Read the model definition and answer for the solid it produces. Units are mm, in the model's axes. Give positions to 0.01 mm unless a question says otherwise; leave off trailing zeros. Loops run counter-clockwise (first coordinate to the right, second up) from the corner with the lowest first, then second, coordinate; pieces in that order, holes last. Notation, with made-up numbers: (2, 76.5) -> (51, 76.5) arc R26 ccw to (51, 100.5) -> close; hole circle Ø5 at (-0.75, -32.75). An arc over 180 degrees is marked (long way). Answer as CSV lines item,"result". Start each with the question number.
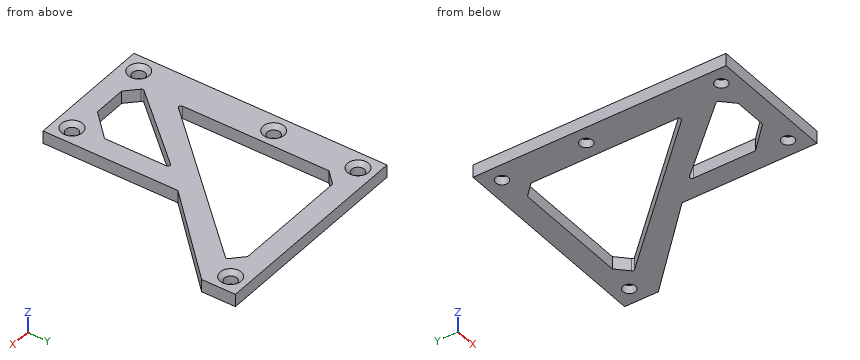
```python
from build123d import *

# Parameters (mm, degrees)
PAD_DEPTH    = 3
SKETCH001_R  = 1.5
POCKET_DEPTH = 5
FILLET_R     = 0.5
FILLET001_R  = 0.5
CHAMFER_SIZE = 1


with BuildPart() as part:
    # Sketch → Pad (new body)
    with BuildSketch(Plane.XY):
        Polygon((0, 0), (0, -60), (8, -60), (30, -60), (30, -28), (50, -8), (50, 0), align=None)
        Polygon((8, -8), (11, -5), (39, -5), (42, -8), (8, -44), align=None, mode=Mode.SUBTRACT)
        Polygon((8, -52), (25, -33), (25, -49), (19, -55), (11, -55), align=None, mode=Mode.SUBTRACT)
    extrude(amount=PAD_DEPTH)

    # Sketch001 (on Face19 of Pad) → Pocket (cut)
    with BuildSketch(Plane.XY.offset(3)):
        with Locations((4, -4)):
            Circle(SKETCH001_R)
        with Locations((46, -4)):
            Circle(SKETCH001_R)
        with Locations((4, -24)):
            Circle(SKETCH001_R)
        with Locations((4, -56)):
            Circle(SKETCH001_R)
        with Locations((26, -56)):
            Circle(SKETCH001_R)
    extrude(amount=-POCKET_DEPTH, mode=Mode.SUBTRACT)

    # Fillet
    fillet_edges = [part.edges().sort_by_distance(p)[0] for p in [
        (8, -44, 1.5),
        (25, -33, 1.5),
    ]]
    fillet(fillet_edges, radius=FILLET_R)

    # Fillet001
    fillet001_edges = [part.edges().sort_by_distance(p)[0] for p in [
        (8, -52, 1.5),
        (42, -8, 1.5),
    ]]
    fillet(fillet001_edges, radius=FILLET001_R)

    # Chamfer
    chamfer_edges = [part.edges().sort_by_distance(p)[0] for p in [
        (2.5, -4, 3),
        (2.5, -24, 3),
        (2.5, -56, 3),
        (24.5, -56, 3),
        (44.5, -4, 3),
    ]]
    chamfer(chamfer_edges, length=CHAMFER_SIZE)


solid = part.part
```
(1) Find section A-A on x = 4. Write down the section's boundary in (y, z), then the cut area to 3 significant figures.
(2) Find section C-C on y = -29. Write down the section's boundary in (x, z).
(3) Find section D-D on z = 2.45. Write down the section's boundary in (x, y), then the cut area to 3 significant figures.
(4) Find section B-B on x = 26. Write down the section's boundary in (y, z), then the cut area to 3 significant figures.
(5) Each of these flat-tipped pins is pushed along its axis until it touches: P1, Ø0.9, axis at y = -21, z = 1.5, coming from the +X side; P2, Ø1.5, axis at y = -49, z = 1, coming from the +X side. Where does it stop, or does it pass through?
(6) Find the intervals of material crossed by line 1 along Y through (x, z) = (4, 1.55); line 2 along X through (y, z) = (-3, 1.8); line 3 along Y through (x, z) = (9, 1.15), in increasing order. Write a range as from..to.
Answer block:
1,outline,"(-60, 0) -> (-57.5, 0) -> (-57.5, 2) -> (-58.5, 3) -> (-60, 3) -> close; (-54.5, 0) -> (-25.5, 0) -> (-25.5, 2) -> (-26.5, 3) -> (-53.5, 3) -> (-54.5, 2) -> close; (-22.5, 0) -> (-5.5, 0) -> (-5.5, 2) -> (-6.5, 3) -> (-21.5, 3) -> (-22.5, 2) -> close; (-2.5, 0) -> (0, 0) -> (0, 3) -> (-1.5, 3) -> (-2.5, 2) -> close"
1,area,"150 mm2"
2,outline,"(0, 0) -> (8, 0) -> (8, 3) -> (0, 3) -> close; (22.17, 0) -> (30, 0) -> (30, 3) -> (22.17, 3) -> close"
3,outline,"(0, -60) -> (30, -60) -> (30, -28) -> (50, -8) -> (50, 0) -> (0, 0) -> close; hole circle Ø3.9 at (4, -56); hole circle Ø3.9 at (4, -24); hole circle Ø3.9 at (4, -4); hole (8, -42.74) arc R0.5 ccw to (8.86, -43.09) -> (41.67, -8.35) arc R0.5 ccw to (41.66, -7.66) -> (39, -5) -> (11, -5) -> (8, -8) -> close; hole (8.32, -51.65) arc R0.5 ccw to (8.33, -52.33) -> (11, -55) -> (19, -55) -> (25, -49) -> (25, -34.31) arc R0.5 ccw to (24.13, -33.98) -> close; hole circle Ø3.9 at (26, -56); hole circle Ø3.9 at (46, -4)"
3,area,"1,210 mm2"
4,outline,"(-60, 0) -> (-57.5, 0) -> (-57.5, 2) -> (-58.5, 3) -> (-60, 3) -> close; (-54.5, 0) -> (-24.94, 0) -> (-24.94, 3) -> (-53.5, 3) -> (-54.5, 2) -> close; (-5, 0) -> (0, 0) -> (0, 3) -> (-5, 3) -> close"
4,area,"110 mm2"
5,P1,"stops at x = 37.45"
5,P2,"stops at x = 30"
6,line 1,"y = -60..-57.5, -54.5..-25.5, -22.5..-5.5, -2.5..0"
6,line 2,"x = 0..2.88, 5.12..44.88, 47.12..50"
6,line 3,"y = -60..-53, -50.88..-42.94, -7..0"
